from build123d import *

# Parameters (mm, degrees)
F2_R = 0.5


with BuildPart() as f1:
    # F0 (on Top) → F1 (revolve)
    with BuildSketch(Plane.XY):
        Polygon((2.9, -2), (0, -2), (0, -65.7), (4.5, -65.7), (4.5, -70), (10.6, -70), (10.6, -2), (11.5, -2), (11.5, -1), (10.4, 0), (2.9, 0), align=None)
    revolve(axis=Axis((0, -33.85, 0), (0, -1, 0)))

    # F2
    f2_edges = [f1.edges().sort_by_distance(p)[0] for p in [
        (-10.6, -70, 0),
        (-4.5, -70, 0),
    ]]
    fillet(f2_edges, radius=F2_R)


solid = f1.part
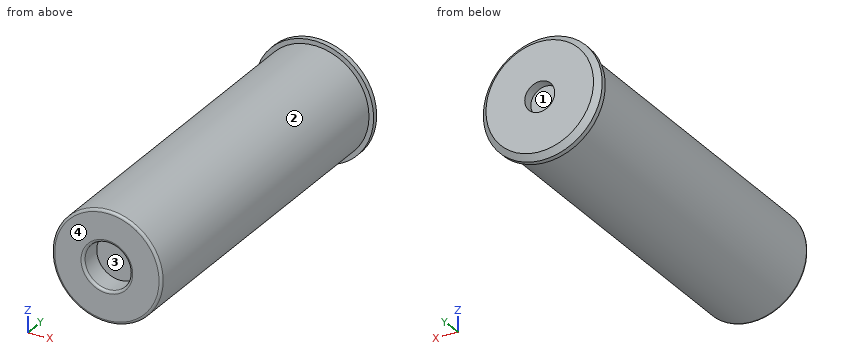
For this review, take the finished solid that the model builds, in its own axes (mm). Face numbers are marked on the shaded views. Give positions to 0.01 mm unless a question says otherwise; leave off trailing zeros. Loops run counter-clockwise (first coordinate to the right, second up) from the corner with the lowest first, then second, coordinate; pieces in that order, holes last. Notation, with made-up numbers: M 45.25,57.25 L 80.25,57.25 A17 cw 80.25,88.25 Z; hole C 65,12 d11. An arc over 180 degrees is marked long. Put each result on its own line as item: value. Start each with the question number.
(1) The part is to be moulded in two halves that separate along X. For the marked faces 1, 2, 3 and 4, say which applies: +X half, -X half, draft (parallel to the pull), parting line (faces both ways), or undercut.
(2) For pin 1 (6.5 mm diameter, centred on x = 0, z = 0, fed in from -Y); pin 2 (10.5 mm diameter, centred on x = 0, z = 0, fed in from -Y); pin 3 (5 mm diameter, centred on x = 7, y = -16, fed in from +Z); pin 4 (10 mm diameter, centred on x = 2, y = -33, fed in from +Z), all flat-tipped, find the tip position at first contact; note any pin that passes through.
(3) Add section B-B, the plane x = 0. Write out the cut boundary in (y, z), then the cut area to 3 significant figures.
(4) Wall thickness on L1, parallel to Z at x = 0, y = -67.7; L2, parallel to Z at x = 0, y = -1.05; L3, parallel to Y at x = 0.5, z = -1: over which ranges is each line inside the solid? List them lowest first.
(5) Add section A-A, the plane z = 0. Write out the cut boundary in (x, y), then the cut area to 3 significant figures.
(6) Add section C-C, the plane y = -56.5. Write out the cut boundary in (x, z), then the cut area to 3 significant figures.
Result:
1. face 1: undercut
1. face 2: parting line
1. face 3: undercut
1. face 4: draft
2. pin 1: stops at y = -65.7
2. pin 2: stops at y = -70
2. pin 3: stops at z = 9.6
2. pin 4: stops at z = 10.6
3. outline: M -70,-10.1 A0.5 ccw -69.5,-10.6 L -2,-10.6 L -2,-11.5 L -1,-11.5 L 0,-10.4 L 0,-2.9 L -2,-2.9 L -2,2.9 L 0,2.9 L 0,10.4 L -1,11.5 L -2,11.5 L -2,10.6 L -69.5,10.6 A0.5 ccw -70,10.1 L -70,5 A0.5 ccw -69.5,4.5 L -65.7,4.5 L -65.7,-4.5 L -69.5,-4.5 A0.5 ccw -70,-5 Z
3. area: 1,440 mm^2
4. L1: z = -10.6 to -4.5, 4.5 to 10.6
4. L2: z = -11.5 to -2.9, 2.9 to 11.5
4. L3: y = -65.7 to -2
5. outline: M -11.5,-2 L -10.6,-2 L -10.6,-69.5 A0.5 ccw -10.1,-70 L -5,-70 A0.5 ccw -4.5,-69.5 L -4.5,-65.7 L 4.5,-65.7 L 4.5,-69.5 A0.5 ccw 5,-70 L 10.1,-70 A0.5 ccw 10.6,-69.5 L 10.6,-2 L 11.5,-2 L 11.5,-1 L 10.4,0 L 2.9,0 L 2.9,-2 L -2.9,-2 L -2.9,0 L -10.4,0 L -11.5,-1 Z
5. area: 1,440 mm^2
6. outline: C 0,0 d21.2
6. area: 353 mm^2
